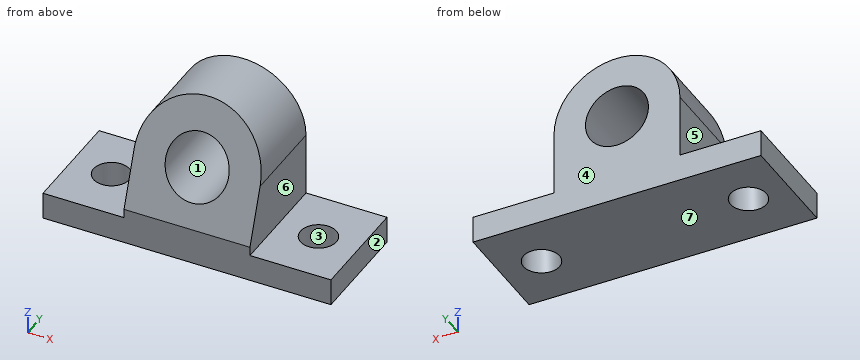
from build123d import *

# Parameters (mm, degrees)
SKETCH_W        = 160
SKETCH_H        = 60
PAD_DEPTH       = 15
SKETCH001_R     = 10
POCKET_DEPTH    = 15.001
SKETCH002_R     = 17.5
PAD001_DEPTH    = 30
POCKET001_DEPTH = 115.001


with BuildPart() as pocket:
    # Sketch → Pad (new body)
    with BuildSketch(Plane.XY):
        Rectangle(SKETCH_W, SKETCH_H)
    extrude(amount=PAD_DEPTH)

    # Sketch001 → Pocket (cut, through all)
    with BuildSketch(Plane.XY.offset(15)):
        with Locations((-57.5, 0)):
            Circle(SKETCH001_R)
        with Locations((57.5, 0)):
            Circle(SKETCH001_R)
    extrude(amount=-POCKET_DEPTH, mode=Mode.SUBTRACT)


with BuildPart() as pocket001:
    # Sketch002 → Pad001 (new body, symmetric)
    with BuildSketch(Plane.XZ):
        with BuildLine():
            ThreePointArc((35, 50), (0, 85), (-35, 50))
            Line((-35, 0), (-35, 50))
            Line((-35, 0), (35, 0))
            Line((35, 0), (35, 50))
        make_face()
        with Locations((0, 50)):
            Circle(SKETCH002_R, mode=Mode.SUBTRACT)
    extrude(amount=PAD001_DEPTH, both=True)

    # Fusion: union Pocket
    add(pocket.part)

    # Sketch003 → Pocket001 (cut, through all)
    with BuildSketch(Plane.YZ.offset(35)):
        Polygon((-30, 15), (-30, 95), (-2.638389, 95.17541), (-30, 20), align=None)
    extrude(amount=-POCKET001_DEPTH, mode=Mode.SUBTRACT)


solid = pocket001.part
Geometry check sheet. Reference: the model listing, model coordinates, mm. Face numbers are marked on the shaded views. A direction names the side the tool comes from. Give positions to 0.01 mm unless a question says otherwise; leave off trailing zeros. Write each loop counter-clockwise with the first axis right and the second up, starting at its lowest first coordinate (ties: lowest second). Pieces come first, ordered by that corner, then holes. Notation, with made-up numbers: (29.25, 63.25) - (87.25, 63.25) arc R36 ccw to (87.25, 98.25) - close; hole circle Ø6 at (66.5, 64.25). An arc over 180 degrees is marked (long way). Put each result on its own line as item: value.
1. Draft check along X on the marked faces 1, 2, 3 and 4. Enter one of: +X half, -X half, draft (parallel to the pull), parting line (faces both ways), or undercut.
Ans:
face 1: undercut
face 2: +X half
face 3: undercut
face 4: draft
2. Go/stop test with flat-tipped pins: pin 1 (17.5 mm diameter, centred on y = -12, z = 31, fed in from +X); pin 2 (6 mm diameter, centred on y = -11, z = 62.5, fed in from -X); pin 3 (8 mm diameter, centred on x = -7.5, z = 31, fed in from -Y); pin 4 (23 mm diameter, centred on x = -57.5, y = 0, fed in from -Z). Record where each tip stops, or that it passes through.
Ans:
pin 1: stops at x = 35
pin 2: stops at x = -33.69
pin 3: stops at y = -27.45
pin 4: stops at z = 0
3. Sectioned sample at B-B, the plane x = 57.5. Enter the section's corners in (y, z), plus the area to 3 significant figures.
Ans:
outline: (-30, 0) - (-10, 0) - (-10, 15) - (-30, 15) - close; (10, 0) - (30, 0) - (30, 15) - (10, 15) - close
area: 600 mm²
4. Thickness scan on line 1 (X direction, y = -4, z = 50); line 2 (Y direction, x = 57.5, z = 8.5); line 3 (Z direction, x = 0, y = 0). Record the ranges inside material, lowest first.
Ans:
line 1: x = -35 to -17.5, 17.5 to 35
line 2: y = -30 to -10, 10 to 30
line 3: z = 0 to 32.5, 67.5 to 85
5. Sectioned sample at D-D, the plane y = 7.5. Enter the section's corners in (x, z), plus the area to 3 significant figures.
Ans:
outline: (-80, 0) - (-64.11, 0) - (-64.11, 15) - (-80, 15) - close; (-50.89, 0) - (50.89, 0) - (50.89, 15) - (35, 15) - (35, 50) arc R35 ccw to (-35, 50) - (-35, 15) - (-50.89, 15) - close; (64.11, 0) - (80, 0) - (80, 15) - (64.11, 15) - close; hole circle Ø35 at (0, 50)
area: 5,420 mm²
6. Sectioned sample at C-C, the plane z = 56.5. Enter the section's corners in (x, y).
Ans:
outline: (-34.39, -16.72) - (-16.25, -16.72) - (-16.25, 30) - (-34.39, 30) - close; (16.25, -16.72) - (34.39, -16.72) - (34.39, 30) - (16.25, 30) - close
7. Sectioned sample at A-A, the plane y = 0. Enter the section's corners in (x, z), plus the area to 3 significant figures.
Ans:
outline: (-80, 0) - (-67.5, 0) - (-67.5, 15) - (-80, 15) - close; (-47.5, 0) - (47.5, 0) - (47.5, 15) - (35, 15) - (35, 50) arc R35 ccw to (-35, 50) - (-35, 15) - (-47.5, 15) - close; (67.5, 0) - (80, 0) - (80, 15) - (67.5, 15) - close; hole circle Ø35 at (0, 50)
area: 5,210 mm²
8. Set-up check for the marked faces 5, 6 and 7: record each of +Z, -Z, +X, -X, +Y, -Y from which the full face is reachable in a straight line by a thin tool's end or side.
Ans:
face 5: +Z, -X, +Y, -Y
face 6: +Z, +X, +Y, -Y
face 7: -Z, +X, -X, +Y, -Y
